Drawing for the job (mm, zero at the part's lowest x, y, z). A direction names the side the tool comes from. Coordinates: 2 decimals unless noted, no trailing zeros. Write each loop counter-clockwise with the first axis right and the second up, starting at its lowest first coordinate (ties: lowest second). Pieces come first, ordered by that corner, then holes. Notation, with made-up numbers: M 63.25,71 L 82.25,71 A26 cw 82.25,107 Z; hole C 56,27 d11. An arc over 180 degrees is marked long. Put each result on its own line as item: value. Start each with the question number.
Q1. Drill centre lines: line 1 along X through (y, z) = (10, 11); line 2 along Z through (x, y) = (11.25, 16.5); line 3 along Z through (x, y) = (9.75, 23). Where is each one in solid material? Low to high.
Q2. Which spindle directions (+Z, -Z, +X, -X, +Y, -Y) get a long thin tool onto all of the face, cutting with end or side? Do the marked faces 4, 5, 6, 7 and 8. Say none if no direction does.
Q3. Cut at B-B (z = 11). Write the cut outline in (x, y), then the cut area to 3 significant figures.
Q4. Cut at D-D (x = 16). Write the cut outline in (y, z).
Q5. Cut at A-A (y = 23). Write the cut outline in (x, z).
Q6. Pull direction X, two halves, no side cores. Call the marked faces 1, 2 and 3: pulls with the +X half, pulls with the -X half, needs draft (parallel to the pull), parting line crosses it, or undercut.
Q7. Cut at C-C (x = 12.5). Write the cut outline in (y, z).
Q8. Drop flat-ended pins along their axis: pin 1 (7 mm diameter, centred on x = 16.5, z = 11, fed in from +Y); pin 2 (11.5 mm diameter, centred on y = 23, z = 11, fed in from -X). Give the stop position or say it passes through.
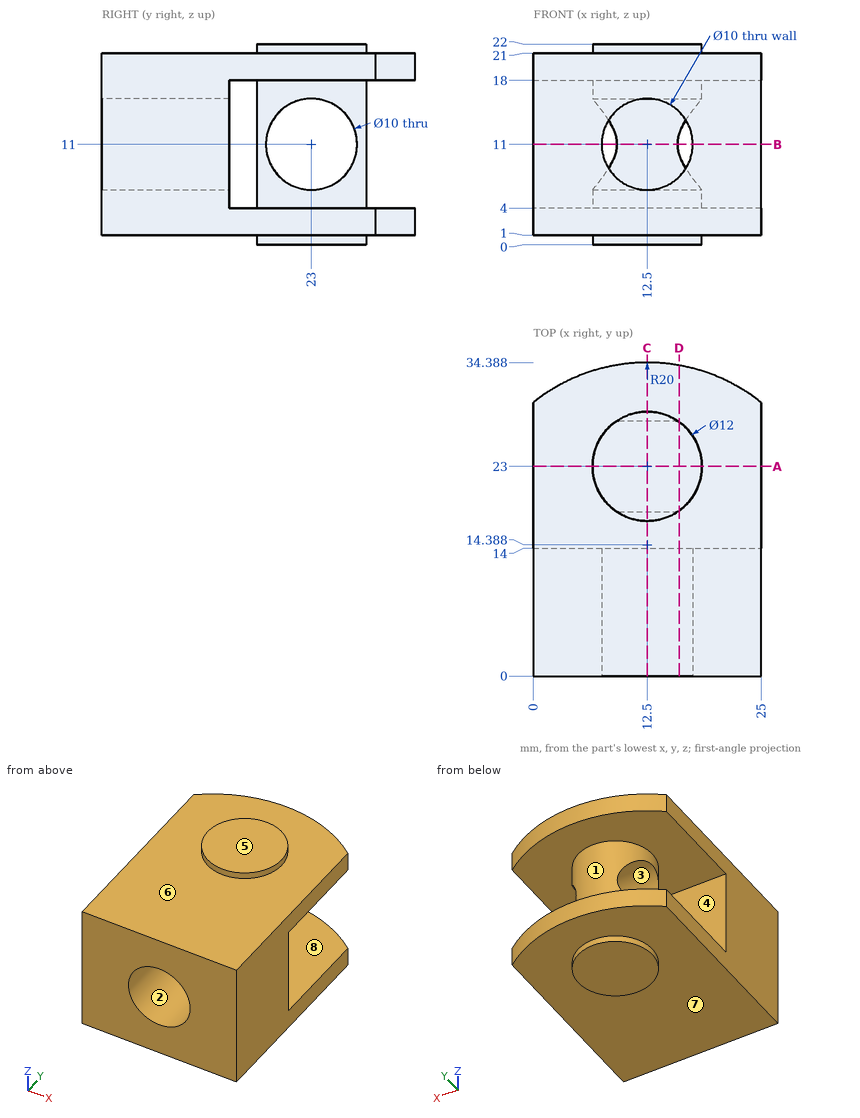
Computed values:
1. line 1: 0 to 7.5, 17.5 to 25
1. line 2: 1 to 4, 18 to 21
1. line 3: 0 to 6, 16 to 22
2. face 4: +X, -X
2. face 5: +Z, +X, -X, +Y, -Y
2. face 6: +Z
2. face 7: -Z
2. face 8: none
3. outline: M 0,0 L 7.5,0 L 7.5,14 L 0,14 Z; M 9.18,18 A6 ccw 15.82,18 Z; M 9.18,28 L 15.82,28 A6 ccw Z; M 17.5,0 L 25,0 L 25,14 L 17.5,14 Z
3. area: 219 mm2
4. outline: M 0,1 L 18.13,1 L 18.13,0 L 27.87,0 L 27.87,1 L 34.08,1 L 34.08,4 L 27.87,4 L 27.87,9.88 A5 cw 18.13,9.88 L 18.13,4 L 14,4 L 14,7.43 L 0,7.43 Z; M 0,14.57 L 14,14.57 L 14,18 L 18.13,18 L 18.13,12.12 A5 cw 27.87,12.12 L 27.87,18 L 34.08,18 L 34.08,21 L 27.87,21 L 27.87,22 L 18.13,22 L 18.13,21 L 0,21 Z
5. outline: M 0,1 L 6.5,1 L 6.5,0 L 18.5,0 L 18.5,1 L 25,1 L 25,4 L 18.5,4 L 18.5,6 L 6.5,6 L 6.5,4 L 0,4 Z; M 0,18 L 6.5,18 L 6.5,16 L 18.5,16 L 18.5,18 L 25,18 L 25,21 L 18.5,21 L 18.5,22 L 6.5,22 L 6.5,21 L 0,21 Z
6. face 1: parting line crosses it
6. face 2: undercut
6. face 3: needs draft
7. outline: M 0,1 L 17,1 L 17,0 L 29,0 L 29,1 L 34.39,1 L 34.39,4 L 29,4 L 29,18 L 34.39,18 L 34.39,21 L 29,21 L 29,22 L 17,22 L 17,21 L 0,21 L 0,16 L 14,16 L 14,18 L 17,18 L 17,4 L 14,4 L 14,6 L 0,6 Z; hole C 23,11 d10
8. pin 1: y = 28.98
8. pin 2: x = 6.5
